Here's the drawing with two shaded views (mm, measured from the low corner). I have some questions. Round coordinates to 2 decimals unless told otherwise and drop trailing zeros. Write each loop counter-clockwise with the first axis right and the second up, starting at its lowest first coordinate (ties: lowest second). Pieces come first, ordered by that corner, then holes. Notation, with made-up numbers: M 43,52.5 L 66,52.5 A21 ccw 66,86.5 Z; hole C 81.25,-35 d2. An arc over 180 degrees is marked long. Write item = value, one per line. Start each with the question number.
(1) I want a section at C-C (z = 38). List the corners of the cut face in (x, y) for me, and give its area (3 significant figures).
(2) I want a section at B-B (y = 25.4). List the corners of the cut face in (x, z) for me, and give its area (3 significant figures).
(3) I want a section at D-D (x = 31.75). List the corners of the cut face in (y, z) for me.
(4) I need wall thicknesses on line 1 along Z through (x, y) = (30, 45.5); line 2 along Z through (x, y) = (6.5, 4); line 3 along X through (y, z) = (28, 23). Which ranges of each line are inside material? Lowest first, please.
(5) I want a section at A-A (x = 57.15). List the corners of the cut face in (y, z) for me (3 decimals), and give its area (3 significant figures).
(6) If we mould it in two halves opening along Y, with no side actions, what happens to the marked faces 1, 2 and 3? For each: released by +Y, released by -Y, zero draft, split by the parting line, or undercut.
(7) Will these pins go through, and if not, where does the flat tip stop? pin 1 Ø1.5 at (x, z) = (35, 57.5) entering from +Y; pin 2 Ø8 at (x, y) = (39.5, 8.5) entering from +Z; pin 3 Ø15 at (x, y) = (21.5, 18.5) entering from -Z.
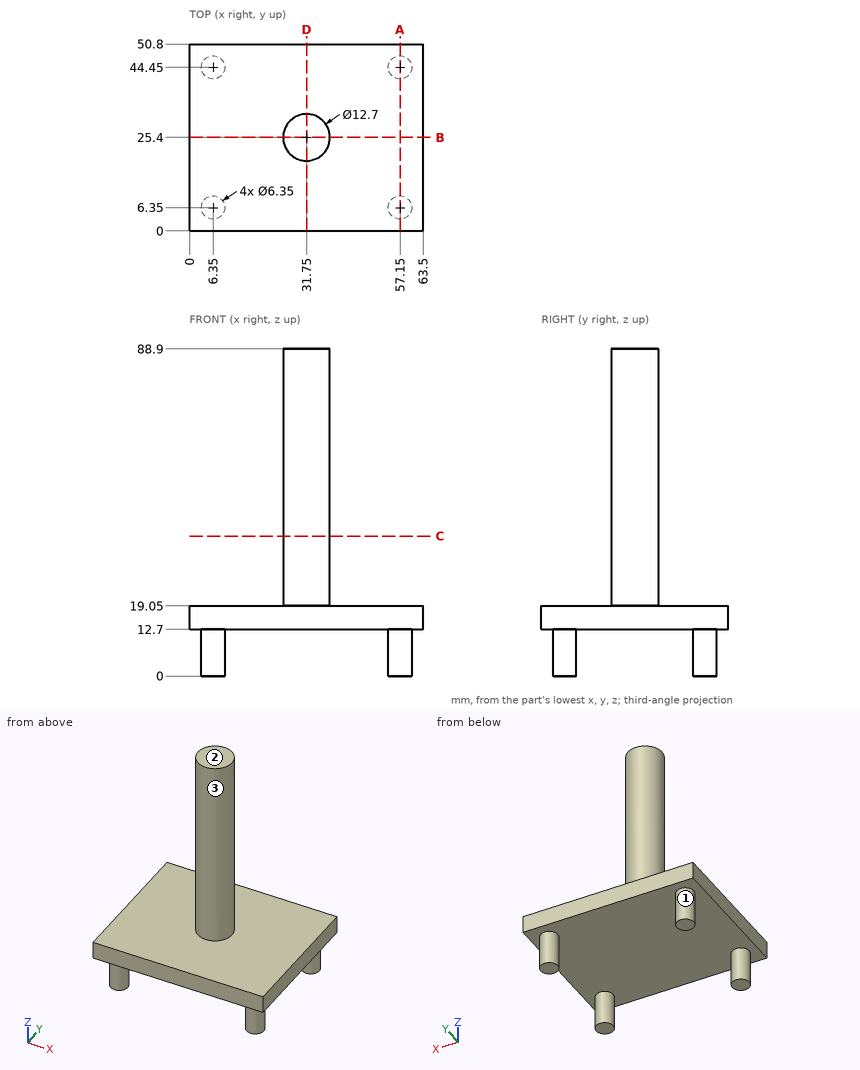
Returned:
q1.outline = C 31.75,25.4 d12.7
q1.area = 127 mm²
q2.outline = M 0,12.7 L 63.5,12.7 L 63.5,19.05 L 38.1,19.05 L 38.1,88.9 L 25.4,88.9 L 25.4,19.05 L 0,19.05 Z
q2.area = 1,290 mm²
q3.outline = M 0,12.7 L 50.8,12.7 L 50.8,19.05 L 31.75,19.05 L 31.75,88.9 L 19.05,88.9 L 19.05,19.05 L 0,19.05 Z
q4.line_1 = 12.7 to 19.05
q4.line_2 = 0 to 19.05
q4.line_3 = 25.96 to 37.54
q5.outline = M 0,12.7 L 3.175,12.7 L 3.175,0 L 9.525,0 L 9.525,12.7 L 41.275,12.7 L 41.275,0 L 47.625,0 L 47.625,12.7 L 50.8,12.7 L 50.8,19.05 L 0,19.05 Z
q5.area = 484 mm²
q6.face_1 = undercut
q6.face_2 = zero draft
q6.face_3 = split by the parting line
q7.pin_1 = 31.24
q7.pin_2 = 19.05
q7.pin_3 = 12.7
